Job drawing, mm, ordinate dimensions from the low corner. One solid piece. A direction names the side the tool comes from. Give positions to 0.01 mm unless a question says otherwise; leave off trailing zeros. Write each loop counter-clockwise with the first axis right and the second up, starting at its lowest first coordinate (ties: lowest second). Pieces come first, ordered by that corner, then holes. Notation, with made-up numbers: (84, 51.25) -> (120, 51.25) arc R22 ccw to (120, 67.25) -> close; hole circle Ø6 at (20.5, 15.5). An arc over 180 degrees is marked (long way). Put each result on its own line as item: value. Start each with the question number.
Item 1: Slice it at A-A, the plane x = 89.5. List the corners of the cut face in (y, z), plus the area to 3 significant figures.
Item 2: Slice it at B-B, the plane y = 41. List the corners of the cut face in (x, z).
Item 3: Slice it at C-C, the plane x = 47.5. List the corners of the cut face in (y, z), plus the area to 3 significant figures.
Item 4: Drill centre lines: line 1 along X through (y, z) = (4, 16); line 2 along Y through (x, z) = (3.5, 7); line 3 along Z through (x, y) = (6, 17.5). Where is each one in solid material? Low to high.
Item 5: Flat gauge pins, fed straight in: pin 1 Ø1.8 at (x, y) = (3.5, 68) entering from -Z; pin 2 Ø5 at (x, y) = (46, 22) entering from +Z. Where does each tip first touch, or does it go through?
Item 6: Tool access for the marked faces 1 and 2: list every direction of +Z, -Z, +X, -X, +Y, -Y with a clear straight run to the whole face (end or side of a thin tool).
Item 7: Two-plate mould, pull along Y, no slides. Class the marked faces 3, 4, 5 and 6: pulls with the +Y half, pulls with the -Y half, needs draft (parallel to the pull), parting line crosses it, or undercut.
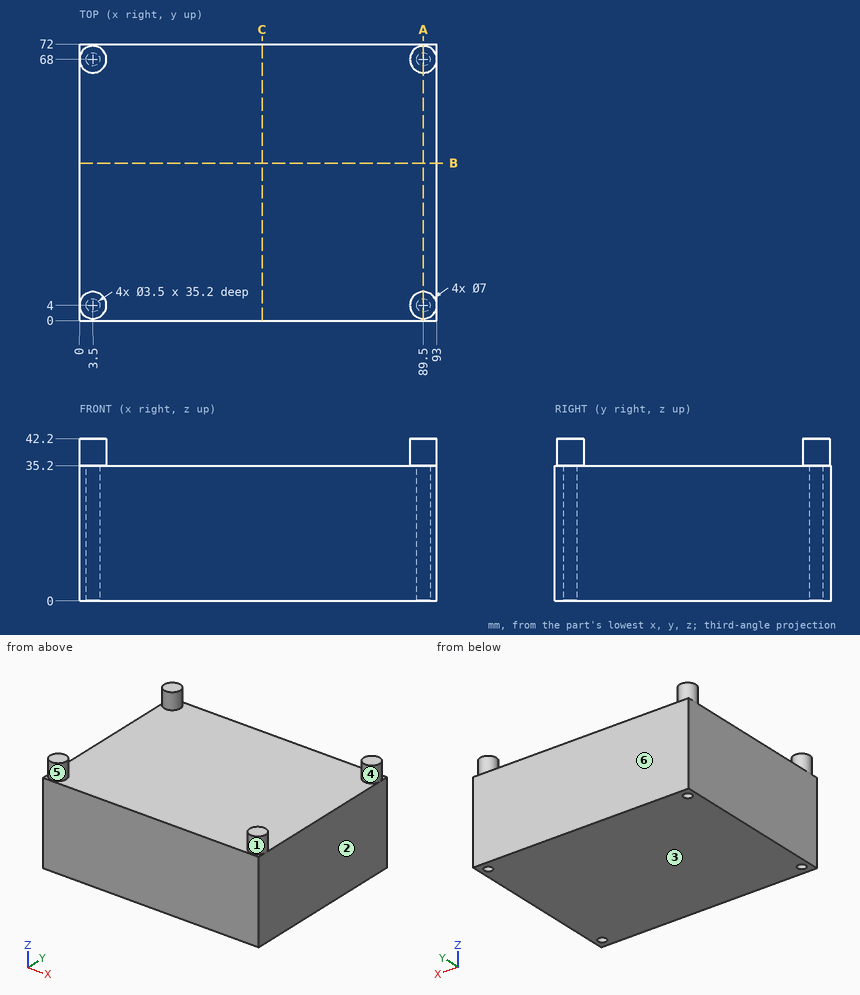
Values follow:
1. outline: (0, 0) -> (2.25, 0) -> (2.25, 35.2) -> (5.75, 35.2) -> (5.75, 0) -> (66.25, 0) -> (66.25, 35.2) -> (69.75, 35.2) -> (69.75, 0) -> (72, 0) -> (72, 35.2) -> (71.5, 35.2) -> (71.5, 42.2) -> (64.5, 42.2) -> (64.5, 35.2) -> (7.5, 35.2) -> (7.5, 42.2) -> (0.5, 42.2) -> (0.5, 35.2) -> (0, 35.2) -> close
1. area: 2,390 mm2
2. outline: (0, 0) -> (93, 0) -> (93, 35.2) -> (0, 35.2) -> close
3. outline: (0, 0) -> (72, 0) -> (72, 35.2) -> (0, 35.2) -> close
3. area: 2,530 mm2
4. line 1: 0 to 1.75, 5.25 to 87.75, 91.25 to 93
4. line 2: 0 to 2.25, 5.75 to 66.25, 69.75 to 72
4. line 3: 0 to 35.2
5. pin 1: z = 35.2
5. pin 2: z = 35.2
6. face 1: +Z
6. face 2: +Z, -Z, +X, +Y, -Y
7. face 3: needs draft
7. face 4: undercut
7. face 5: undercut
7. face 6: pulls with the +Y half
